```python
from build123d import *

# Parameters (mm, degrees)
SKETCH2_W           = 14.3
SKETCH2_H           = 14.3
BOSS_EXTRUDE1_DEPTH = 5.6
CUT_EXTRUDE2_DEPTH  = 17.5
LPATTERN1_COUNT     = 5
LPATTERN1_PITCH     = 2.25
LPATTERN1_COL_COUNT = 4
LPATTERN1_COL_PITCH = 2.25


with BuildPart() as part:
    # Sketch2 → Boss-Extrude1 (new body)
    with BuildSketch(Plane(origin=(-2.586863131, -15.699309697, 9.787522701), x_dir=(0.9597170343404154, -0.24447167145746004, -0.13848038074627608), z_dir=(0.13848038074627628, 0.8404180176603395, -0.5239472680912))):
        with Locations((20.198681335, -0.426078635)):
            Rectangle(SKETCH2_W, SKETCH2_H)
    extrude(amount=BOSS_EXTRUDE1_DEPTH)

    # Sketch3 → Cut-Extrude2 (cut)
    with BuildSketch(Plane(origin=(-1.643808295, -3.252120737, -5.650904665), x_dir=(-0.9696564349576585, 0.12194238719709705, 0.21188782964077374), z_dir=(-0.24447167145746004, -0.4836643024316157, -0.8404180176603393))):
        with BuildLine():
            Line((-17.670554194, -16.169704918), (-17.199268448, -19.435878481))
            ThreePointArc((-17.199268448, -19.435878481), (-17.121093331, -19.567484364), (-16.972755762, -19.605265621))
            Line((-16.972755762, -19.605265621), (-15.93351872, -19.455311066))
            ThreePointArc((-15.93351872, -19.455311066), (-15.801912836, -19.377135948), (-15.764131579, -19.22879838))
            Line((-15.764131579, -19.22879838), (-16.235417325, -15.962624817))
            ThreePointArc((-16.235417325, -15.962624817), (-16.159854811, -15.665949681), (-15.896643044, -15.509599446))
            Line((-15.896643044, -15.509599446), (-18.123579565, -15.830930637))
            ThreePointArc((-18.123579565, -15.830930637), (-17.826904429, -15.906493151), (-17.670554194, -16.169704918))
        make_face()
    cut_extrude2 = extrude(amount=-CUT_EXTRUDE2_DEPTH, mode=Mode.SUBTRACT)

    # LPattern1: Cut-Extrude2 ×5
    with Locations(*[Vector(0.9597170343404154, -0.24447167145746015, -0.138480380746276) * (i * LPATTERN1_PITCH) for i in range(1, LPATTERN1_COUNT)]):
        add(cut_extrude2, mode=Mode.SUBTRACT)

    # LPattern1 col: Cut-Extrude2 ×4
    with Locations(*[Vector(-0.9597170343404154, 0.2444716714574598, 0.13848038074627622) * (i * LPATTERN1_COL_PITCH) for i in range(1, LPATTERN1_COL_COUNT)]):
        add(cut_extrude2, mode=Mode.SUBTRACT)


solid = part.part
```
Input: part model. Units: mm. Frame: model coordinates. A direction names the side the tool comes from. Coordinates: 2 decimals unless noted, no trailing zeros. Use a Markdown table: item, result. Add a question column.
1) Line query: L1, parallel to Z at x = 17, y = -15.75; L2, parallel to Z at x = 11, y = -22; L3, parallel to Y at x = 16.25, z = 5.25. Output: solid intervals per line, ascending. Write a range as from..to.
2) Pin query (flat end, axial travel): P1, Ø8, axis at x = 18.5, z = -0.5, coming from the +Y side; P2, Ø4, axis at x = 14.5, y = -19.5, coming from the -Z side; P3, Ø4, axis at x = 21, y = -14, coming from the -Z side. Return the tip coordinate at first contact, or that it passes through.
3) Draft query along X for faces 5 (the flat face through (11.72, -17.68, 7.15)), 6 (the flat face through (16.782, -20.455, 7.278)). Return one class per face: +X half, -X half, draft (parallel to the pull), parting line (faces both ways), or undercut.
4) Set-up query: faces 1 (the flat face through (15.354, -22.068, 0.233)), 2 (the cylindrical face through (19.722, -19.666, 5.968)), 3 (the flat face through (12.67, -16.28, 6.07)), 4 (the flat face through (20.359, -19.878, 5.905)). Return all of +Z, -Z, +X, -X, +Y, -Y with unobstructed straight access to the full face (end or side cutting, diameter ignored); none if empty.
Answer below:
| question | item | result |
|---|---|---|
| 1 | L1 | 11.64..13.13 |
| 1 | L2 | 1.46..3.27 |
| 1 | L3 | -21.63..-19.6 |
| 2 | P1 | y = -16.35 |
| 2 | P2 | z = -1.6 |
| 2 | P3 | z = 4.94 |
| 3 | face 5 | undercut |
| 3 | face 6 | -X half |
| 4 | face 1 | -Z, -X, -Y |
| 4 | face 2 | -Z |
| 4 | face 3 | +Y |
| 4 | face 4 | none |
